```python
from build123d import *

# Parameters (mm, degrees)
SKETCH1_R                   = 110
SKETCH1_R_2                 = 4.7625
BOSS_EXTRUDE1_DEPTH         = 2.6
SKETCH2_R                   = 2.15
CUT_EXTRUDE3_DEPTH          = 6.2
CIRPATTERN1_COUNT           = 2
CIRPATTERN2_COUNT           = 2
CIRPATTERN2_ANGLE           = 60
CIRPATTERN2_COPY_1_SKETCH_R = 2.15
CIRPATTERN2_COPY_1_DEPTH    = 6.2
CUT_EXTRUDE5_DEPTH          = 6.2
SKETCH11_R                  = 3
SKETCH11_W                  = 25
SKETCH11_H                  = 5.2
CUT_EXTRUDE24_DEPTH         = 6.2
CUT_EXTRUDE25_DEPTH         = 6.2
CUT_EXTRUDE26_DEPTH         = 6.2


with BuildPart() as part:
    # Sketch1 → Boss-Extrude1 (new body, symmetric)
    with BuildSketch(Plane.XY):
        Circle(SKETCH1_R)
        Circle(SKETCH1_R_2, mode=Mode.SUBTRACT)
        Polygon((-4.7625, 40), (-2.2625, 40), (-2.2625, 48), (0.7375, 48), (0.7375, 93), (-19.2625, 93), (-19.2625, 40), (-16.7625, 40), align=None, mode=Mode.SUBTRACT)
        Polygon((4.7625, -40), (2.2625, -40), (2.2625, -48), (-0.7375, -48), (-0.7375, -93), (19.2625, -93), (19.2625, -40), (16.7625, -40), align=None, mode=Mode.SUBTRACT)
    extrude(amount=BOSS_EXTRUDE1_DEPTH, both=True)

    # Sketch2 → Cut-Extrude3 (cut, through all)
    with BuildSketch(Plane.XY.offset(2.6)):
        with Locations((11.7625, -97.435)):
            Circle(SKETCH2_R)
        with BuildLine():
            Line((-10.7375, -82.808492409), (-10.7375, -101.8725))
            Line((-10.7375, -101.8725), (9.2625, -101.8725))
            Line((9.2625, -101.8725), (29.2625, -101.8725))
            Line((29.2625, -101.8725), (29.2625, -82.808492409))
            Line((29.2625, -82.808492409), (36.2625, -82.808492409))
            Line((36.2625, -82.808492409), (46.112001713, -99.868329805))
            ThreePointArc((46.112001713, -99.868329805), (0, -110), (-46.112001713, -99.868329805))
            Line((-46.112001713, -99.868329805), (-36.2625, -82.808492409))
            Line((-36.2625, -82.808492409), (-10.7375, -82.808492409))
        make_face()
    cut_extrude3 = extrude(amount=-CUT_EXTRUDE3_DEPTH, mode=Mode.SUBTRACT)

    # CirPattern1: Cut-Extrude3 ×2 about axis
    cirpattern1_axis = Axis((0, 0, 0), (0, 0, 1))
    for i in range(1, CIRPATTERN1_COUNT):
        add(cut_extrude3.rotate(cirpattern1_axis, i * 360 / CIRPATTERN1_COUNT), mode=Mode.SUBTRACT)

    # CirPattern2: Cut-Extrude3 ×2 about axis
    cirpattern2_axis = Axis((0, 0, 0), (0, 0, 1))
    for i in range(1, CIRPATTERN2_COUNT):
        add(cut_extrude3.rotate(cirpattern2_axis, i * CIRPATTERN2_ANGLE / (CIRPATTERN2_COUNT - 1)), mode=Mode.SUBTRACT)

    # CirPattern2 copy 1 sketch → CirPattern2 copy 1 (cut, through all)
    with BuildSketch(Plane(origin=(0, 0, 2.6), x_dir=(-0.5, -0.866025404, 0), z_dir=(0, 0, 1))):
        with Locations((11.7625, -97.435)):
            Circle(CIRPATTERN2_COPY_1_SKETCH_R)
        with BuildLine():
            Line((-10.7375, -82.808492409), (-10.7375, -101.8725))
            Line((-10.7375, -101.8725), (9.2625, -101.8725))
            Line((9.2625, -101.8725), (29.2625, -101.8725))
            Line((29.2625, -101.8725), (29.2625, -82.808492409))
            Line((29.2625, -82.808492409), (36.2625, -82.808492409))
            Line((36.2625, -82.808492409), (46.112001713, -99.868329805))
            ThreePointArc((46.112001713, -99.868329805), (0, -110), (-46.112001713, -99.868329805))
            Line((-46.112001713, -99.868329805), (-36.2625, -82.808492409))
            Line((-36.2625, -82.808492409), (-10.7375, -82.808492409))
        make_face()
    extrude(amount=-CIRPATTERN2_COPY_1_DEPTH, mode=Mode.SUBTRACT)

    # Sketch5 → Cut-Extrude5 (cut, through all)
    with BuildSketch(Plane.XY.offset(2.6)):
        with BuildLine():
            Line((89.845508076, 10), (53.583008076, 72.808492409))
            Line((53.583008076, 72.808492409), (63.432509788, 89.868329805))
            ThreePointArc((63.432509788, 89.868329805), (95.262794416, 55), (109.544511501, 10))
            Line((109.544511501, 10), (89.845508076, 10))
        make_face()
        with BuildLine():
            Line((-89.845508076, -10), (-53.583008076, -72.808492409))
            Line((-53.583008076, -72.808492409), (-63.432509788, -89.868329805))
            ThreePointArc((-63.432509788, -89.868329805), (-95.262794416, -55), (-109.544511501, -10))
            Line((-109.544511501, -10), (-89.845508076, -10))
        make_face()
    extrude(amount=-CUT_EXTRUDE5_DEPTH, mode=Mode.SUBTRACT)

    # Sketch11 → Cut-Extrude24 (cut, through all)
    with BuildSketch(Plane.XY.offset(2.6)):
        with Locations((45.241826211, -53.255843194)):
            Circle(SKETCH11_R)
        with Locations((-23.5, -65.808492409)):
            Circle(SKETCH11_R)
        with Locations((-68.741826211, -12.552649216)):
            Circle(SKETCH11_R)
        with Locations((-45.241826211, 53.255843194)):
            Circle(SKETCH11_R)
        with Locations((23.5, 65.808492409)):
            Circle(SKETCH11_R)
        with Locations((68.741826211, 12.552649216)):
            Circle(SKETCH11_R)
        Polygon((-1.7375, -48), (23.2625, -48), (23.2625, -42.8), (19.2625, -42.8), (2.2625, -42.8), (-1.7375, -42.8), align=None)
        Polygon((-42.437969382, -22.495280861), (-29.937969382, -44.145915956), (-25.434637282, -41.545915956), (-37.934637282, -19.895280861), align=None)
        Polygon((-20.7625, -33.025), (-16.7625, -33.025), (-4.7625, -33.025), (-0.7625, -33.025), (-0.7625, -38.225), (-20.7625, -38.225), align=None)
        Polygon((-38.98173896, 1.468352446), (-36.98173896, -1.995749169), (-30.98173896, -12.388054014), (-28.98173896, -15.85215563), (-33.48507106, -18.45215563), (-43.48507106, -1.131647554), align=None)
        Polygon((-40.700469382, 25.504719139), (-53.200469382, 3.854084044), (-48.697137282, 1.254084044), (-36.197137282, 22.904719139), align=None)
        Polygon((-18.21923896, 34.493352446), (-20.21923896, 31.029250831), (-26.21923896, 20.636945986), (-28.21923896, 17.17284437), (-32.72257106, 19.77284437), (-22.72257106, 37.093352446), align=None)
        with Locations((-10.7625, 45.4)):
            Rectangle(SKETCH11_W, SKETCH11_H)
        Polygon((42.437969382, 22.495280861), (29.937969382, 44.145915956), (25.434637282, 41.545915956), (37.934637282, 19.895280861), align=None)
        Polygon((20.7625, 33.025), (16.7625, 33.025), (4.7625, 33.025), (0.7625, 33.025), (0.7625, 38.225), (20.7625, 38.225), align=None)
        Polygon((40.700469382, -25.504719139), (53.200469382, -3.854084044), (48.697137282, -1.254084044), (36.197137282, -22.904719139), align=None)
        Polygon((38.98173896, -1.468352446), (36.98173896, 1.995749169), (30.98173896, 12.388054014), (28.98173896, 15.85215563), (33.48507106, 18.45215563), (43.48507106, 1.131647554), align=None)
        Polygon((18.21923896, -34.493352446), (20.21923896, -31.029250831), (26.21923896, -20.636945986), (28.21923896, -17.17284437), (32.72257106, -19.77284437), (22.72257106, -37.093352446), align=None)
    extrude(amount=-CUT_EXTRUDE24_DEPTH, mode=Mode.SUBTRACT)

    # Sketch12 → Cut-Extrude25 (cut, through all)
    with BuildSketch(Plane.XY.offset(2.6)):
        Polygon((-37, -64.08587988), (-34.74833395, -65.38587988), (-39.74833395, -74.046133918), (-44.25166605, -71.446133918), (-39.25166605, -62.78587988), align=None)
        Polygon((-51, -88.334591186), (-48.74833395, -89.634591186), (-43.74833395, -80.974337148), (-48.25166605, -78.374337148), (-53.25166605, -87.034591186), align=None)
        Polygon((-74, 0), (-74, -2.6), (-84, -2.6), (-84, 2.6), (-74, 2.6), align=None)
        Polygon((-102, 0), (-102, -2.6), (-92, -2.6), (-92, 2.6), (-102, 2.6), align=None)
        Polygon((-37, 64.08587988), (-39.25166605, 62.78587988), (-44.25166605, 71.446133918), (-39.74833395, 74.046133918), (-34.74833395, 65.38587988), align=None)
        Polygon((-51, 88.334591186), (-53.25166605, 87.034591186), (-48.25166605, 78.374337148), (-43.74833395, 80.974337148), (-48.74833395, 89.634591186), align=None)
        Polygon((37, 64.08587988), (34.74833395, 65.38587988), (39.74833395, 74.046133918), (44.25166605, 71.446133918), (39.25166605, 62.78587988), align=None)
        Polygon((51, 88.334591186), (48.74833395, 89.634591186), (43.74833395, 80.974337148), (48.25166605, 78.374337148), (53.25166605, 87.034591186), align=None)
        Polygon((74, 0), (74, 2.6), (84, 2.6), (84, -2.6), (74, -2.6), align=None)
        Polygon((102, 0), (102, 2.6), (92, 2.6), (92, -2.6), (102, -2.6), align=None)
        Polygon((37, -64.08587988), (39.25166605, -62.78587988), (44.25166605, -71.446133918), (39.74833395, -74.046133918), (34.74833395, -65.38587988), align=None)
        Polygon((51, -88.334591186), (53.25166605, -87.034591186), (48.25166605, -78.374337148), (43.74833395, -80.974337148), (48.74833395, -89.634591186), align=None)
    extrude(amount=-CUT_EXTRUDE25_DEPTH, mode=Mode.SUBTRACT)

    # Sketch13 → Cut-Extrude26 (cut, through all)
    with BuildSketch(Plane.XY.offset(2.6)):
        Polygon((-86.345508076, 16.062177826), (-66.345508076, 50.703193978), (-76.345508076, 67.59574596), (-92.560678517, 57.996740162), (-113.304387557, 22.067582168), align=None)
        Polygon((66.345508076, -50.703193978), (83.10535709, -79.014856047), (116.539469578, -32.259052148), (108.045386829, -17.910378712), (86.345508076, -16.062177826), align=None)
    extrude(amount=-CUT_EXTRUDE26_DEPTH, mode=Mode.SUBTRACT)


solid = part.part
```
Source: CAD feature listing. Evaluate the final solid. Frame: model axes, mm. A direction names the side the tool comes from. Round coordinates to 2 decimals unless told otherwise and drop trailing zeros. Use a Markdown table: item, result. Add a question column.
1. Contact query for flat-ended pins moving along their axis: pin 1 (2.5 mm diameter, centred on y = 77, z = 0, fed in from +X); pin 2 (1 mm diameter, centred on y = -9.5, z = -1.5, fed in from -X); pin 3 (2 mm diameter, centred on y = -41, z = 0.5, fed in from -X) (3 decimals). Output: stop coordinate, or through.
2. Cut plane A-A, the plane z = -0.4. State how many separate pieces and enclosed holes the cut face has, and give its area (3 significant figures).
3. Set-up query: faces 1 (the flat face through (-9, 101.872, 0)), 2 (the flat face through (-20.5, 35.81, 0.04)), 3 (the flat face through (24, 82.808, 0)). Return all of +Z, -Z, +X, -X, +Y, -Y with unobstructed straight access to the full face (end or side cutting, diameter ignored); none if empty.
4. Pull-direction query (X, two-part tool) for faces 4 (the flat face through (100, -10, 0)), 5 (the flat face through (51.032, 88.316, 0.036)); classes: +X half, -X half, draft (parallel to the pull), parting line (faces both ways), or undercut.
5. Ray query, line 1 along Y through (x, z) = (12, 1.2) (1 decimal); line 2 along Y through (x, z) = (-0.5, -1.6); line 3 along Y through (x, z) = (-17.5, -0.7) (1 decimal). Return the intervals inside material, ascending. Write a range as [from, to].
Solution:
| question | item | result |
|---|---|---|
| 1 | pin 1 | stops at x = 56.72 |
| 1 | pin 2 | stops at x = -109.63 |
| 1 | pin 3 | stops at x = -72.525 |
| 2 | separate pieces | 1 |
| 2 | enclosed holes | 33 |
| 2 | area | 23,100 mm2 |
| 3 | face 1 | +Z, -Z, +X, -X, +Y |
| 3 | face 2 | +Z, -Z |
| 3 | face 3 | +Z, -Z, +Y |
| 4 | face 4 | draft |
| 4 | face 5 | undercut |
| 5 | line 1 | y = [-101.9, -99.6], [-95.3, -93], [-40, 33], [38.2, 82.8] |
| 5 | line 2 | y = [-101.87, -93], [-42.8, -4.74], [4.74, 42.8], [93, 101.87] |
| 5 | line 3 | y = [-82.8, -38.2], [-33, 40], [93, 101.9] |
